from build123d import *

# Parameters (mm, degrees)
BOSS_EXTRUDE1_DEPTH = 145
BOSS_EXTRUDE2_DEPTH = 7


with BuildPart() as part:
    # Sketch1 → Boss-Extrude1 (new body)
    with BuildSketch(Plane.XY):
        Polygon((2.1, 1.3), (5.5, 1.3), (5.5, 0), (0, 0), (0, 14.057025137), (21.040065237, 32.34687481), (84.759934763, 32.34687481), (105.8, 14.057025137), (105.8, 0), (100.3, 0), (100.3, 1.3), (103.7, 1.3), (103.7, 13.1), (83.974776936, 30.24687481), (21.825223064, 30.24687481), (2.1, 13.1), align=None)
    extrude(amount=BOSS_EXTRUDE1_DEPTH)

    # Sketch2 → Boss-Extrude2 (add)
    with BuildSketch(Plane(origin=(0, 0, 0), x_dir=(-1, 0, 0), z_dir=(0, 0, -1))):
        Polygon((-2.1, 0), (0, 0), (0, 14.057025137), (-21.040065237, 32.34687481), (-84.759934763, 32.34687481), (-105.8, 14.057025137), (-105.8, 0), (-103.7, 0), (-103.7, 13.1), (-83.974776936, 30.24687481), (-21.825223064, 30.24687481), (-2.1, 13.1), align=None)
    extrude(amount=BOSS_EXTRUDE2_DEPTH)


solid = part.part
The listing builds one solid part. Answer for the finished solid, in the listing's coordinates (mm). A direction names the side the tool comes from. Round coordinates to 2 decimals unless told otherwise and drop trailing zeros. Write each loop counter-clockwise with the first axis right and the second up, starting at its lowest first coordinate (ties: lowest second). Pieces come first, ordered by that corner, then holes. Notation, with made-up numbers: (80, 11.25) - (134, 11.25) arc R24 ccw to (134, 22.25) - close; hole circle Ø3 at (13, 31). An arc over 180 degrees is marked (long way). Use a Markdown table: item, result. Add a question column.
1. A tool of negligible diameter and unlimited length cuts with its end or side. For faces 1 (the face through (102, 1.3, 71)), 2 (the face through (52, 32.347, 70)), from which of +Z, -Z, +X, -X, +Y, -Y can it reach the whole face along a straight path? Write none if from no direction.
2. Consider line 1 (X direction, y = 9.5, z = 35); line 2 (Y direction, x = 25, z = 3); line 3 (X direction, y = 25.5, z = 19.5). Determine where each line is inside the solid, lowest interval first.
3. The part is cut by section D-D (x = 68). Write down the section's boundary in (y, z).
4. The part is cut by section A-A (y = 5). Write down the section's boundary in (x, z), and give its area (3 significant figures).
5. Flat-ended cylindrical pins translate along their axes: P1, Ø8, axis at x = 94.5, y = 25.5, coming from the -Z side; P2, Ø1, axis at y = 22.5, z = 115.5, coming from the +X side; P3, Ø1.4, axis at x = 4, y = 0.5, coming from the -Z side; P4, Ø1.7, axis at x = 101.5, z = 58, coming from the +Y side. Find the tip coordinate at first contact, or state that the pin passes through.
6. The part is cut by section B-B (z = 14.5). Write down the section's boundary in (x, y).
7. The part is cut by section C-C (y = 26). Write down the section's boundary in (x, z).
8. For a pull along X with two mould halves and no side action, classify faces 3 (the face through (61, 31, 145)), 4 (the face through (53, 30.247, 70)), 5 (the face through (105.8, 7, 70)), 6 (the face through (0, 7, 70)) as +X half, -X half, draft (parallel to the pull), parting line (faces both ways), or undercut.
Reported:
| question | item | result |
|---|---|---|
| 1 | face 1 | +Z, -Z |
| 1 | face 2 | +Z, -Z, +X, -X, +Y |
| 2 | line 1 | 0 to 2.1, 103.7 to 105.8 |
| 2 | line 2 | 30.25 to 32.35 |
| 2 | line 3 | 13.16 to 16.36, 89.44 to 92.64 |
| 3 | outline | (30.25, -7) - (32.35, -7) - (32.35, 145) - (30.25, 145) - close |
| 4 | outline | (0, -7) - (2.1, -7) - (2.1, 145) - (0, 145) - close; (103.7, -7) - (105.8, -7) - (105.8, 145) - (103.7, 145) - close |
| 4 | area | 638 mm^2 |
| 5 | P1 | z = -7 |
| 5 | P2 | x = 96.66 |
| 5 | P3 | z = 0 |
| 5 | P4 | y = 18.53 |
| 6 | outline | (0, 0) - (5.5, 0) - (5.5, 1.3) - (2.1, 1.3) - (2.1, 13.1) - (21.83, 30.25) - (83.97, 30.25) - (103.7, 13.1) - (103.7, 1.3) - (100.3, 1.3) - (100.3, 0) - (105.8, 0) - (105.8, 14.06) - (84.76, 32.35) - (21.04, 32.35) - (0, 14.06) - close |
| 7 | outline | (13.74, -7) - (16.94, -7) - (16.94, 145) - (13.74, 145) - close; (88.86, -7) - (92.06, -7) - (92.06, 145) - (88.86, 145) - close |
| 8 | face 3 | draft |
| 8 | face 4 | undercut |
| 8 | face 5 | +X half |
| 8 | face 6 | -X half |
